The listing builds one solid part. Answer for the finished solid, in the listing's coordinates (mm). A direction names the side the tool comes from. Coordinates: 2 decimals unless noted, no trailing zeros. Order: outer loops, then holes, each group sorted by start corner. A loop starts at its lowest first (then second) coordinate and runs counter-clockwise, first axis right, second up. Notation, with made-up numbers: (58, 44.5) -> (64, 44.5) arc R22 cw to (64, 62.5) -> close; hole circle Ø10 at (83, 47.5). An arc over 180 degrees is marked (long way). Answer in a Markdown table with one row per item.
Autodesk Inventor part; units mm, degrees
ref_plane "YZ Plane" through (0, 0, 0) normal (1, 0, 0) x (0, 1, 0)
ref_plane "XZ Plane" through (0, 0, 0) normal (0, 1, 0) x (-1, 0, 0)
ref_plane "XY Plane" through (0, 0, 0) normal (0, 0, 1) x (1, 0, 0)
sketch "Sketch1" plane through (0, 0, 0) normal (1, 0, 0) x (0, 1, 0)
  line L0 (0, 0) -> (11.4, 0)
  line L1 (11.4, 0) -> (11.4, -12.1)
  line L2 (11.4, -12.1) -> (0, -12.1)
  line L3 (0, -12.1) -> (0, 0)
  arc A0 (11.4, -2.9512) -> (11.4, -9.1488) centre (12.8006, -6.05) ccw
  point P0 (3.5, -5)
  dimension "d0" = 11.4
  dimension "d1" = 12.1
  dimension "d2" = 6.1976
  dimension "d3" = 2.9512
  dimension "d29" = 2
extrude "Extrusion1" add sketch "Sketch1" along normal blind 6.35
extrude "Extrusion2" add sketch "Sketch1" against normal blind 12.7 contours L1 A0
sketch "Sketch3" plane through (0, 0, 0) normal (-1, 0, 0) x (0, 0, 1)
  line L0 (0, 11.4) -> (0, 0)
  line L1 (0, 0) -> (-12.1, 0)
  point P0 (-6.05, 5.7)
  dimension "d19" = 12.1
  dimension "d20" = 6.05
  dimension "d30" = 11.4
  dimension "d31" = 5.7
hole "Hole2" at (0, 5.7, -6.05) direction (1, 0, 0) diameter 4 end through all
sketch "Sketch9" plane through (0, 0, -12.1) normal (0, 0, -1) x (-1, 0, 0)
  line L0 (-6.35, 0) -> (-6.35, 11.4)
  line L1 (0, 0) -> (0, 11.4)
  line L2 (-6.35, 11.4) -> (0, 11.4)
  line L3 (0, 11.4) -> (0, 5.7)
  line L4 (0, 5.7) -> (-6.35, 5.7)
  line L5 (-6.35, 5.7) -> (-6.35, 11.4)
  dimension "d70" = 11.4
  dimension "d71" = 5.7
extrude "Extrusion10" add sketch "Sketch9" along normal blind 3.175
sketch "Sketch10" plane through (0, 0, -15.275) normal (0, 0, -1) x (-1, 0, 0)
  circle A0 centre (-3.175, 8.55) radius 1.9939
  line L0 (-6.35, 11.4) -> (-6.35, 5.7)
  line L1 (0, 11.4) -> (-6.35, 11.4)
  point P0 (0, 0)
  dimension "d74" = 6.35
  dimension "d75" = 5.7
  dimension "d76" = 2.85
  dimension "d77" = 3.175
  dimension "d80" = 3.9878
extrude "Extrusion11" cut sketch "Sketch10" against normal up to surface (3.175 mm away)
thread "Thread3"
equation "\"d3\" = -0.5 * d2 + 0.5 * d1"
equation "\"d71\" = 0.5 * d70"
equation "\"d76\" = 0.5 * d75"
equation "\"d77\" = 0.5 * d74"
properties part number "end peice for slides"
(1) Flat-ended cylindrical pins translate along their axes: pin 1 (2 mm diameter, centred on x = 3.5, y = 8.5, fed in from -Z); pin 2 (1 mm diameter, centred on x = 2, z = -13.5, fed in from -Y); pin 3 (3 mm diameter, centred on y = 2.5, z = -9.5, fed in from -X); pin 4 (2.5 mm diameter, centred on y = 5.7, z = -6.05, fed in from -X). Find the tip coordinate at first contact, or state that the pin passes through.
Check values:
| item | result |
|---|---|
| pin 1 | z = -12.1 |
| pin 2 | y = 5.7 |
| pin 3 | x = 0 |
| pin 4 | through |
(2) A cutting plane is placed at C-C, the plane x = 3. Determine the outline of the cut face in (y, z) (3 decimals), then the cut area to 3 significant figures.
Check values:
| item | result |
|---|---|
| outline | (0, -12.1) -> (5.7, -12.1) -> (5.7, -15.275) -> (6.564, -15.275) -> (6.564, -12.1) -> (10.536, -12.1) -> (10.536, -15.275) -> (11.4, -15.275) -> (11.4, 0) -> (0, 0) -> close; hole circle Ø4 at (5.7, -6.05) |
| area | 131 mm² |
(3) A cutting plane is placed at B-B, the plane y = 6. Determine the outline of the cut face in (x, z) (3 decimals).
Check values:
| item | result |
|---|---|
| outline | (0, -15.275) -> (6.35, -15.275) -> (6.35, -8.027) -> (0, -8.027) -> close; (0, -4.073) -> (6.35, -4.073) -> (6.35, 0) -> (0, 0) -> close |
(4) Find the intervals of material crossed by line 1 along X through (y, z) = (9, -5.75); line 2 along Y through (x, z) = (3.25, -6.05); line 3 along X through (y, z) = (6.75, -12.5), in increasing order. Write a range as from..to.
Check values:
| item | result |
|---|---|
| line 1 | 0..6.35 |
| line 2 | 0..3.7, 7.7..11.4 |
| line 3 | 0..2.32, 4.03..6.35 |
(5) A cutting plane is placed at A-A, the plane z = -6.05. Determine the outline of the cut face in (x, y), then the cut area to 3 significant figures.
Check values:
| item | result |
|---|---|
| outline | (-12.7, 9.4) -> (0, 9.4) -> (0, 7.7) -> (6.35, 7.7) -> (6.35, 11.4) -> (-12.7, 11.4) -> close; (0, 0) -> (6.35, 0) -> (6.35, 3.7) -> (0, 3.7) -> close |
| area | 72.4 mm² |
(6) A cutting plane is placed at D-D, the plane y = 8.55. Determine the outline of the cut face in (x, z) (3 decimals).
Check values:
| item | result |
|---|---|
| outline | (0, -15.275) -> (1.181, -15.275) -> (1.181, -12.1) -> (5.169, -12.1) -> (5.169, -15.275) -> (6.35, -15.275) -> (6.35, 0) -> (0, 0) -> close |
(7) Which of the six approach directions +Z, -Z, +X, -X, +Y, -Y give full straight-line access (tool end or side, diameter ignored) to faces 1 (the cylindrical face through (2.255, 6.781, -13.71)), 2 (the cylindrical face through (-6.3, 9.4, -6)), 3 (the flat face through (3, 0, -6)), 4 (the flat face through (3, 3, -12.1))?
Check values:
| item | result |
|---|---|
| face 1 | -Z |
| face 2 | -X, -Y |
| face 3 | +Z, -Z, +X, -X, -Y |
| face 4 | -Z, +X, -X, -Y |
(8) For a pull along X with two mould halves and no side action, classify faces 5 (the flat face through (6.35, 4, -8)), 6 (the flat face through (3, 9, -12.1)), 7 (the flat face through (5.34, 8.59, -15.275)) as released by +X, released by -X, zero draft, split by the parting line, or undercut.
Check values:
| item | result |
|---|---|
| face 5 | released by +X |
| face 6 | undercut |
| face 7 | zero draft |
